Check sheet for the drawn part. Datum: minimum x, y, z corner. Units: mm. A direction names the side the tool comes from. Coordinates: 2 decimals unless noted, no trailing zeros. Order: outer loops, then holes, each group sorted by start corner. A loop starts at its lowest first (then second) coordinate and runs counter-clockwise, first axis right, second up. Notation, with made-up numbers: (47.25, 55) -> (83.25, 55) arc R36 ccw to (83.25, 90) -> close; hole circle Ø10 at (74, 27). An arc over 180 degrees is marked (long way). Answer as CSV lines item,"result".
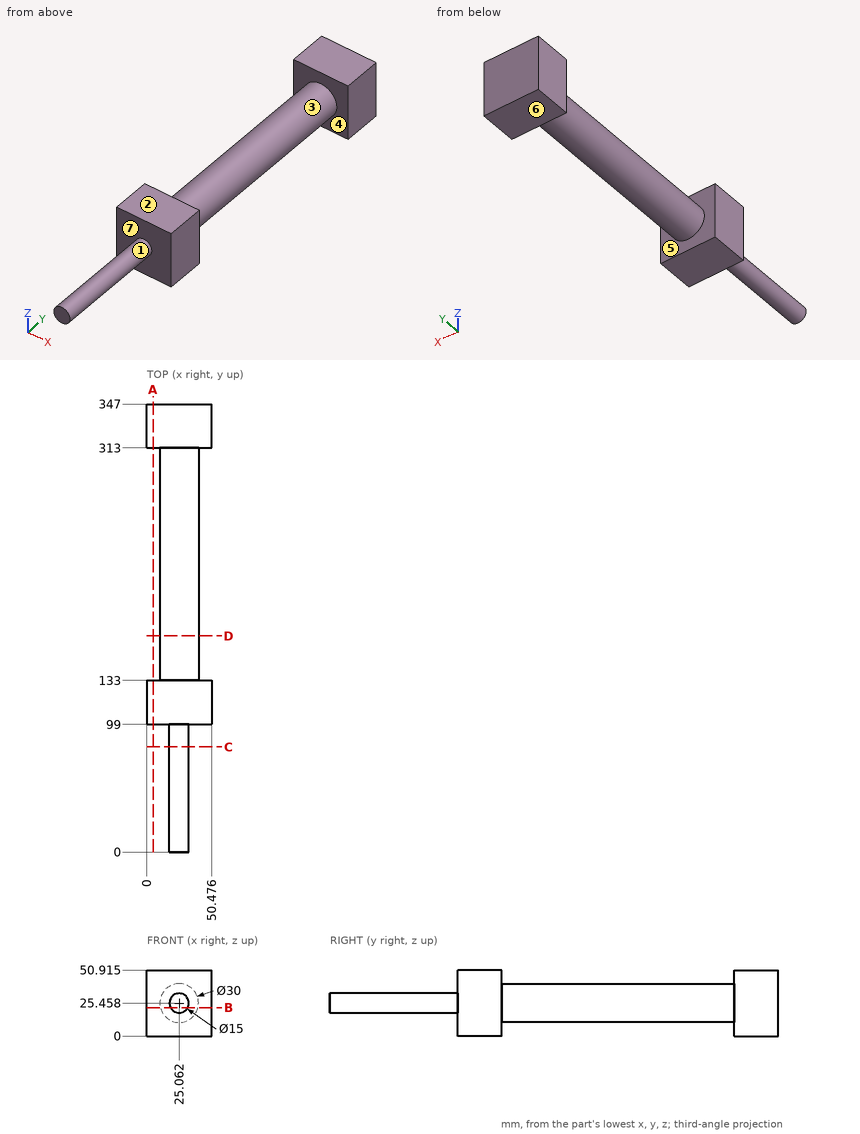
Item 1: Section check A-A, the plane x = 5. Record the boundary of the cut face in (y, z) (1 decimal).
Answer list:
outline,"(99, 0) -> (133, 0) -> (133, 50.9) -> (99, 50.9) -> close; (313, 0) -> (347, 0) -> (347, 50.9) -> (313, 50.9) -> close"
Item 2: Thickness scan on line 1 (Y direction, x = 36, z = 2); line 2 (Y direction, x = 32.5, z = 24); line 3 (X direction, y = 312.5, z = 25.5). Record the ranges inside material, lowest first.
Answer list:
line 1,"99 to 133, 313 to 347"
line 2,"99 to 347"
line 3,"10.06 to 40.06"
Item 3: Tool access check on the marked faces 1, 2 and 3. Record the directions out of +Z, -Z, +X, -X, +Y, -Y that give a thin tool (end or side, any length) a straight path to the whole face; none if there is none.
Answer list:
face 1,"-Y"
face 2,"+Z, +X, -X, +Y, -Y"
face 3,"none"
Item 4: Section check C-C, the plane y = 81.5. Record the boundary of the cut face in (x, z).
Answer list:
outline,"circle Ø15 at (25.06, 25.46)"
Item 5: Release check for a two-part mould opening along Y. For the marked faces 4, 5, 6 and 7 record: +Y half, -Y half, draft (parallel to the pull), parting line (faces both ways), or undercut.
Answer list:
face 4,"undercut"
face 5,"undercut"
face 6,"draft"
face 7,"-Y half"
Item 6: Depth check by flat-ended pin: pin 1 Ø5 at (x, y) = (25.5, 40.5) entering from -Z; pin 2 Ø4 at (y, z) = (203.5, 15.5) entering from -X; pin 3 Ø3 at (y, z) = (286.5, 8) entering from +X; pin 4 Ø12 at (x, z) = (15.5, 11) entering from -Y. Enter the tip coordinate at first touch or a pass-through.
Answer list:
pin 1,"z = 17.96"
pin 2,"x = 12.35"
pin 3,"through"
pin 4,"y = 99"
Item 7: Section check D-D, the plane y = 167.5. Record the boundary of the cut face in (x, z), plus the area to 3 significant figures.
Answer list:
outline,"circle Ø30 at (25.06, 25.46)"
area,"707 mm2"
Item 8: Section check B-B, the plane z = 22. Record the boundary of the cut face in (x, y) (1 decimal), plus the area to 3 significant figures.
Answer list:
outline,"(0, 99) -> (18.4, 99) -> (18.4, 0) -> (31.7, 0) -> (31.7, 99) -> (50.5, 99) -> (50.5, 133) -> (39.7, 133) -> (39.7, 313) -> (50.5, 313) -> (50.5, 347) -> (0, 347) -> (0, 313) -> (10.5, 313) -> (10.5, 133) -> (0, 133) -> close"
area,"10,000 mm2"
